Here's how the part is built. I have some questions about the finished solid (model axes, mm). Give positions to 0.01 mm unless a question says otherwise; leave off trailing zeros. Write each loop counter-clockwise with the first axis right and the second up, starting at its lowest first coordinate (ties: lowest second). Pieces come first, ordered by that corner, then holes. Notation, with made-up numbers: (18.25, -8) -> (31.25, -8) arc R30 ccw to (31.25, 26) -> close; hole circle Ø10 at (-3.75, 18.5). An arc over 180 degrees is marked (long way). Return JSON: item names as keys, results as strings.
from build123d import *

# Parameters (mm, degrees)
F2_DEPTH = 25
F3_SIZE  = 0.5
F4_R     = 1.55
F5_DEPTH = 5


with BuildPart() as f1:
    # F0 (on Right) → F1 (revolve)
    with BuildSketch(Plane.YZ):
        with BuildLine():
            Line((1.5, 0), (7, 0))
            Line((7, 0), (7, 4))
            Line((7, 4), (-8, 4))
            ThreePointArc((-8, 4), (-10.8284271247, 2.8284271247), (-12, 0))
            Line((-12, 0), (-1.5, 0))
            ThreePointArc((-1.5, 0), (0, 1.5), (1.5, 0))
        make_face()
        with BuildLine():
            ThreePointArc((-1.5, 0), (0, -1.5), (1.5, 0))
            Line((1.5, 0), (-1.5, 0))
        make_face()
        with BuildLine():
            Line((-1.5, 0), (1.5, 0))
            ThreePointArc((1.5, 0), (0, 1.5), (-1.5, 0))
        make_face()
    revolve(axis=Axis((0, -2.5, 0), (0, -1, 0)))

    # F0 (on Right) → F2 (cut)
    with BuildSketch(Plane.YZ):
        with BuildLine():
            Line((-1.5, 0), (1.5, 0))
            ThreePointArc((1.5, 0), (0, 1.5), (-1.5, 0))
        make_face()
        with BuildLine():
            ThreePointArc((-1.5, 0), (0, -1.5), (1.5, 0))
            Line((1.5, 0), (-1.5, 0))
        make_face()
    extrude(amount=-F2_DEPTH, mode=Mode.SUBTRACT)

    # F3
    f3_edges = [f1.edges().sort_by_distance(p)[0] for p in [
        (0, 7, -4),
    ]]
    chamfer(f3_edges, length=F3_SIZE)

    # F4 (on face) → F5 (cut)
    with BuildSketch(Plane(origin=(0, 7, 0), x_dir=(-1, 0, 0), z_dir=(0, 1, 0))):
        Circle(F4_R)
    extrude(amount=-F5_DEPTH, mode=Mode.SUBTRACT)


solid = f1.part
1. Suppose I cut it at D-D, the plane y = -9. List the corners of the cut face in (x, z) for me, and give its area (3 significant figures).
Taken from the geometry:
{"outline": "circle Ø7.75 at (0, 0)", "area": "47.1 mm²"}
2. Suppose I cut it at B-B, the plane y = -2.75. List the corners of the cut face in (x, z) for me.
Taken from the geometry:
{"outline": "circle Ø8 at (0, 0)"}
3. If we mould it in two halves opening along Y, with no side actions, what happens to faces 1 (the face through (-1.973, -1.386, 0.575)), 2 (the face through (-0.715, 4.535, -1.375)), 3 (the face through (0, 2, 0))? For each: released by +Y, released by -Y, zero draft, split by the parting line, or undercut.
Taken from the geometry:
{"face 1": "undercut", "face 2": "zero draft", "face 3": "released by +Y"}
4. For pin 1 Ø2 at (y, z) = (2.5, 2) entering from -X; pin 2 Ø1 at (x, y) = (2.5, 2) entering from -Z; pin 3 Ø0.9 at (x, z) = (0.5, -0.5) entering from +Y, each with a flat end and sliding along its axis, tell me the tip position at first contact or that it passes through.
Taken from the geometry:
{"pin 1": "stops at x = -3.87", "pin 2": "stops at z = -3.46", "pin 3": "stops at y = 2"}
5. If I drill on line 1 (Z direction, x = 0, y = 5.85); line 2 (Y direction, x = -3, z = 0.75); line 3 (Y direction, x = -2.7, z = 0), over which ranges is the centre line in solid material (lowest first)? Write a range as [from, to].
Taken from the geometry:
{"line 1": "z = [-4, -1.55], [1.55, 4]", "line 2": "y = [-10.54, -1.3], [1.3, 7]", "line 3": "y = [-10.95, -1.5], [1.5, 7]"}
6. Suppose I cut it at A-A, the plane z = 0. List the corners of the cut face in (x, y) for me, and give its area (3 significant figures).
Taken from the geometry:
{"outline": "(-4, -8) arc R4 ccw to (4, -8) -> (4, 6.5) -> (3.5, 7) -> (1.55, 7) -> (1.55, 2) -> (-1.55, 2) -> (-1.55, 7) -> (-3.5, 7) -> (-4, 6.5) -> (-4, 1.5) -> (0, 1.5) arc R1.5 cw to (0, -1.5) -> (-4, -1.5) -> close", "area": "114 mm²"}
7. Suppose I cut it at C-C, the plane y = 0. List the corners of the cut face in (x, z) for me, and give its area (3 significant figures).
Taken from the geometry:
{"outline": "(-3.71, -1.5) arc R4 ccw (long way) to (-3.71, 1.5) -> (0, 1.5) arc R1.5 cw to (0, -1.5) -> close", "area": "35.0 mm²"}
